Build history of the part. All positions in model axes, mm. Face numbers are marked on the shaded views. A direction names the side the tool comes from. Coordinates: 2 decimals unless noted, no trailing zeros. Order: outer loops, then holes, each group sorted by start corner. A loop starts at its lowest first (then second) coordinate and runs counter-clockwise, first axis right, second up. Notation, with made-up numbers: (80.5, -18) - (110.5, -18) arc R24 cw to (110.5, 17) - close; hole circle Ø9 at (12.5, 75). An arc over 180 degrees is marked (long way). One line per item, written item: value.
from build123d import *

# Parameters (mm, degrees)
CYLINDER003_R     = 1.7
CYLINDER003_DEPTH = 10
CYLINDER002_R     = 1.7
CYLINDER002_DEPTH = 10
BOX003_W          = 8
BOX003_H          = 8
BOX003_DEPTH      = 1.5
CHAMFER001_SIZE   = 0.5
BOX002_W          = 13.5
BOX002_H          = 8
BOX002_DEPTH      = 3
CHAMFER004_SIZE   = 0.4


with BuildPart() as cylinder003:
    # Cylinder003 → Cylinder003 (new body)
    with BuildSketch(Plane(origin=(-4, 11, 0), x_dir=(1, 0, 0), z_dir=(0, 0, 1))):
        Circle(CYLINDER003_R)
    extrude(amount=CYLINDER003_DEPTH)


with BuildPart() as fusion002:
    # Cylinder002 → Cylinder002 (new body)
    with BuildSketch(Plane(origin=(4, 11, 0), x_dir=(1, 0, 0), z_dir=(0, 0, 1))):
        Circle(CYLINDER002_R)
    extrude(amount=CYLINDER002_DEPTH)

    # Fusion002: union Cylinder003
    add(cylinder003.part)


with BuildPart() as chamfer001:
    # Box003 → Box003 (new body)
    with BuildSketch(Plane(origin=(-4, 7, 7.5), x_dir=(1, 0, 0), z_dir=(0, 0, 1))):
        with Locations((4, 4)):
            Rectangle(BOX003_W, BOX003_H)
    extrude(amount=BOX003_DEPTH)

    # Chamfer001
    chamfer001_edges = [chamfer001.edges().sort_by_distance(p)[0] for p in [
        (-4, 11, 7.5),
        (4, 11, 7.5),
    ]]
    chamfer(chamfer001_edges, length=CHAMFER001_SIZE)


with BuildPart() as chamfer004:
    # Box002 → Box002 (new body)
    with BuildSketch(Plane(origin=(-6.75, 7, 5), x_dir=(1, 0, 0), z_dir=(0, 0, 1))):
        with Locations((6.75, 4)):
            Rectangle(BOX002_W, BOX002_H)
    extrude(amount=BOX002_DEPTH)

    # Cut002008023012009006003002006002006002004004003: cut Chamfer001
    add(chamfer001.part, mode=Mode.SUBTRACT)

    # Cut002008023012009006003002006002006002004004004: cut Fusion002
    add(fusion002.part, mode=Mode.SUBTRACT)

    # Chamfer004
    chamfer004_edges = [chamfer004.edges().sort_by_distance(p)[0] for p in [
        (-6.75, 7, 6.5),
        (-6.75, 15, 6.5),
        (6.75, 7, 6.5),
        (5.375, 7, 8),
        (3.75, 7, 7.75),
        (0, 7, 7.5),
        (-3.75, 7, 7.75),
        (-5.375, 7, 8),
        (0, 7, 5),
        (-5.375, 15, 8),
        (6.75, 15, 6.5),
        (5.375, 15, 8),
        (3.75, 15, 7.75),
        (0, 15, 7.5),
        (-3.75, 15, 7.75),
        (0, 15, 5),
    ]]
    chamfer(chamfer004_edges, length=CHAMFER004_SIZE)


solid = chamfer004.part
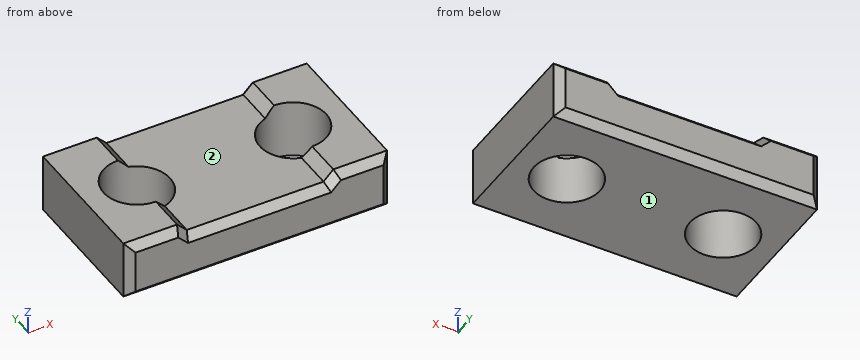
1. Band-saw the part on C-C, the plane x = 4.75. Give the cut face in (y, z), and give its area (3 significant figures).
Values found:
outline: (7, 5.4) - (7.4, 5) - (9.47, 5) - (9.47, 8) - (7.4, 8) - (7, 7.6) - close; (12.53, 5) - (14.6, 5) - (15, 5.4) - (15, 7.6) - (14.6, 8) - (12.53, 8) - close
area: 14.5 mm2
2. 3-axis set-ups, long thin cutter, end or side, ignore diameter. For the marked faces 1 and 2: which of +Z, -Z, +X, -X, +Y, -Y reach the whole face in a straight line?
Values found:
face 1: -Z, +X, -X, +Y, -Y
face 2: +Z, +Y, -Y
3. Band-saw the part on D-D, the plane y = 8.25. Give the cut face in (x, z).
Values found:
outline: (-6.75, 5) - (6.75, 5) - (6.75, 8) - (4, 8) - (3.5, 7.5) - (-3.5, 7.5) - (-4, 8) - (-6.75, 8) - close
4. Flat gauge pins, fed straight in: P1, Ø2.5, axis at x = -4, y = 11, coming from the +Z side; P2, Ø3.5, axis at x = 1, y = 12.5, coming from the +Z side. Where does each tip first touch, or does it go through?
Values found:
P1: passes through
P2: stops at z = 7.5
5. Band-saw the part on B-B, the plane z = 6.85. Give the cut face in (x, y), and give its area (3 significant figures).
Values found:
outline: (-6.75, 7.4) - (-6.35, 7) - (6.35, 7) - (6.75, 7.4) - (6.75, 14.6) - (6.35, 15) - (-6.35, 15) - (-6.75, 14.6) - close; hole circle Ø3.4 at (-4, 11); hole circle Ø3.4 at (4, 11)
area: 89.5 mm2
6. Probe line 1 along Y through (x, z) = (-4, 5.9); line 2 along X through (y, z) = (11, 7.2); line 3 along X through (y, z) = (12, 5.6). List the from-to ranges inside material, lowest first.
Values found:
line 1: y = 7 to 9.3, 12.7 to 15
line 2: x = -6.75 to -5.7, -2.3 to 2.3, 5.7 to 6.75
line 3: x = -6.75 to -5.37, -2.63 to 2.63, 5.37 to 6.75
7. Band-saw the part on A-A, the plane y = 11. Give the cut face in (x, z).
Values found:
outline: (-6.75, 5) - (-5.7, 5) - (-5.7, 8) - (-6.75, 8) - close; (-2.3, 5) - (2.3, 5) - (2.3, 7.5) - (-2.3, 7.5) - close; (5.7, 5) - (6.75, 5) - (6.75, 8) - (5.7, 8) - close
